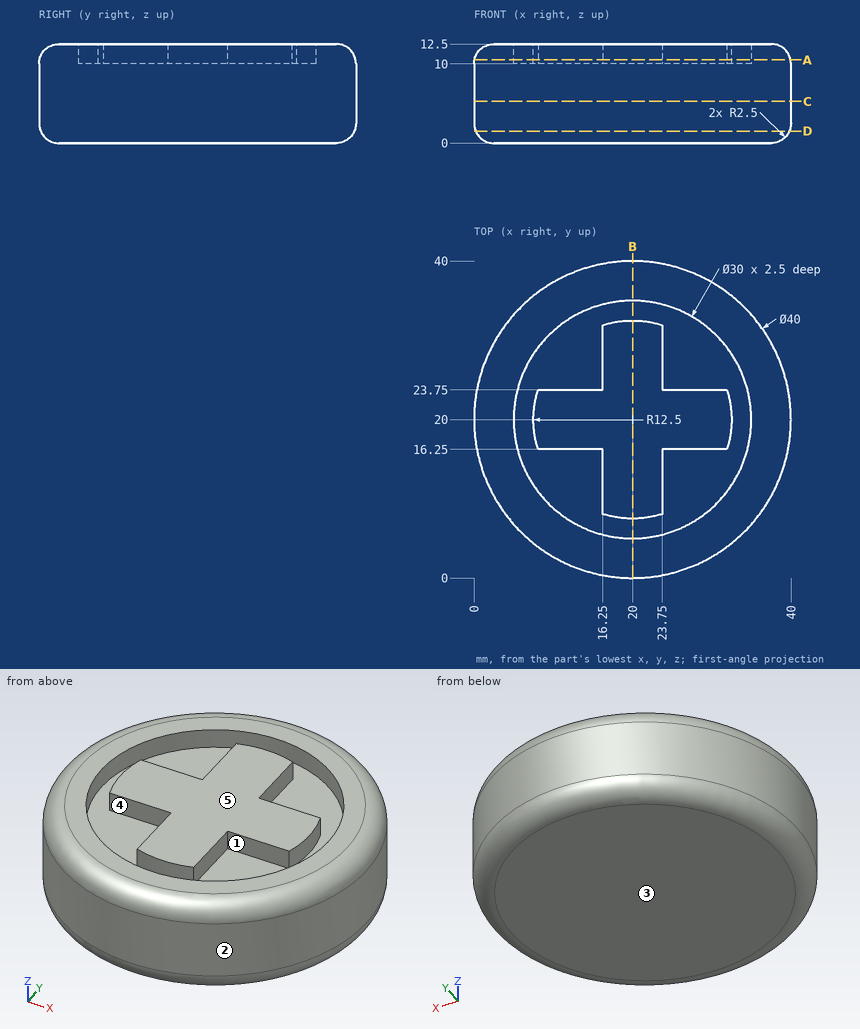
Answer from the drawing. Dimensions are ordinates in mm from the lowest x, y and z of the part. A direction names the side the tool comes from. Round coordinates to 2 decimals unless told otherwise and drop trailing zeros. Write each loop counter-clockwise with the first axis right and the second up, starting at its lowest first coordinate (ties: lowest second). Pieces come first, ordered by that corner, then holes.
1. Given pin 1 Ø3 at (y, z) = (28, 11) entering from -X; pin 2 Ø0.8 at (x, z) = (27.5, 11) entering from +Y; pin 3 Ø3 at (x, z) = (27, 10.5) entering from -Y, each flat-ended and moving along its own axis, determine where each tip first touches the part or whether it passes through.
2. The part is cut by section C-C, the plane z = 5.25. Determine the outline of the cut face in (x, y), then the cut area to 3 significant figures.
3. The part is cut by section D-D, the plane z = 1.5. Determine the outline of the cut face in (x, y), then the cut area to 3 significant figures.
4. The part is cut by section B-B, the plane x = 20. Determine the outline of the cut face in (y, z), then the cut area to 3 significant figures.
5. The part is cut by section A-A, the plane z = 10.5. Determine the outline of the cut face in (x, y).
6. Determine the mould class of the marked faces 1, 2 and 3 for opening direction X: pulls with the +X half, pulls with the -X half, needs draft (parallel to the pull), parting line crosses it, or undercut.
7. Straight lines are drawn through the part: L1, parallel to Y at x = 25, z = 10.25; L2, parallel to Y at x = 20, z = 11.35; L3, parallel to Z at x = 25, y = 37. For each, find the intervals that lie inside material, in ascending order.
8. Which of the six approach directions +Z, -Z, +X, -X, +Y, -Y give full straight-line access (tool end or side, diameter ignored) to the marked faces 4 and 5?
Values:
1. pin 1: stops at x = 1.16
1. pin 2: stops at y = 38.54
1. pin 3: stops at y = 0.79
2. outline: circle Ø40 at (20, 20)
2. area: 1,260 mm2
3. outline: circle Ø39.58 at (20, 20)
3. area: 1,230 mm2
4. outline: (0, 2.5) arc R2.5 ccw to (2.5, 0) - (37.5, 0) arc R2.5 ccw to (40, 2.5) - (40, 10) arc R2.5 ccw to (37.5, 12.5) - (35, 12.5) - (35, 10) - (32.5, 10) - (32.5, 12.5) - (7.5, 12.5) - (7.5, 10) - (5, 10) - (5, 12.5) - (2.5, 12.5) arc R2.5 ccw to (0, 10) - close
4. area: 482 mm2
5. outline: circle Ø39.9 at (20, 20); (8.08, 16.25) - (16.25, 16.25) - (16.25, 8.08) arc R12.5 ccw to (23.75, 8.08) - (23.75, 16.25) - (31.92, 16.25) arc R12.5 ccw to (31.92, 23.75) - (23.75, 23.75) - (23.75, 31.92) arc R12.5 ccw to (16.25, 31.92) - (16.25, 23.75) - (8.08, 23.75) arc R12.5 ccw to start; hole circle Ø30 at (20, 20)
6. face 1: undercut
6. face 2: parting line crosses it
6. face 3: needs draft
7. L1: y = 0.65 to 5.86, 16.25 to 23.75, 34.14 to 39.35
7. L2: y = 0.4 to 5, 7.5 to 32.5, 35 to 39.6
7. L3: z = 0.01 to 12.49
8. face 4: +Z
8. face 5: +Z, +X, -X, +Y, -Y
